The listing builds one solid part. Answer for the finished solid, in the listing's coordinates (mm). A direction names the side the tool comes from. Round coordinates to 2 decimals unless told otherwise and drop trailing zeros. Loops run counter-clockwise (first coordinate to the right, second up) from the corner with the lowest first, then second, coordinate; pieces in that order, holes last. Notation, with made-up numbers: M 62.25,-29 L 119.25,-29 A28 ccw 119.25,-4 Z; hole C 85.5,74 d6. An arc over 180 degrees is marked long. Answer as a JSON object with one key per item and string values.
```python
from build123d import *

# Parameters (mm, degrees)
SKETCH1_R             = 22.225
SKETCH1_R_2           = 20.955
EXTRUDE_THIN1_DEPTH   = 20.32
SKETCH1_R_3           = 14.605
SKETCH1_R_4           = 13.335
EXTRUDE_THIN1_2_DEPTH = 20.32
SKETCH1_3_R           = 8.7757
SKETCH1_3_R_2         = 6.8707
EXTRUDE_THIN2_DEPTH   = 20.32
SKETCH2_W             = 1.27
SKETCH2_H             = 41.91
SKETCH2_W_2           = 41.91
SKETCH2_H_2           = 1.27
EXTRUDE_THIN3_DEPTH   = 20.32
SKETCH1_5_R           = 6.8707
CUT_EXTRUDE1_DEPTH    = 20.32
EXTRUDE_THIN6_DEPTH   = 20.32
CIRPATTERN1_COUNT     = 8


with BuildPart() as part:
    # Sketch1 → Extrude-Thin1 (new body, symmetric)
    with BuildSketch(Plane(origin=(0, 0, 0), x_dir=(0, 0, -1), z_dir=(1, 0, 0))):
        Circle(SKETCH1_R)
        Circle(SKETCH1_R_2, mode=Mode.SUBTRACT)
    extrude(amount=EXTRUDE_THIN1_DEPTH, both=True)



with BuildPart() as body_2:
    # Sketch1 → Extrude-Thin1 2 (new body, symmetric)
    with BuildSketch(Plane(origin=(0, 0, 0), x_dir=(0, 0, -1), z_dir=(1, 0, 0))):
        Circle(SKETCH1_R_3)
        Circle(SKETCH1_R_4, mode=Mode.SUBTRACT)
    extrude(amount=EXTRUDE_THIN1_2_DEPTH, both=True)


with BuildPart() as body_3:
    # Sketch1<3> → Extrude-Thin2 (new body, symmetric)
    with BuildSketch(Plane(origin=(0, 0, 0), x_dir=(0, 0, -1), z_dir=(1, 0, 0))):
        Circle(SKETCH1_3_R)
        Circle(SKETCH1_3_R_2, mode=Mode.SUBTRACT)
    extrude(amount=EXTRUDE_THIN2_DEPTH, both=True)


with BuildPart() as part_1:
    add(part.part)

    add(body_3.part)  # Extrude-Thin3 merges body 3
    # Sketch2 → Extrude-Thin3 (add, symmetric)
    with BuildSketch(Plane(origin=(0, 0, 0), x_dir=(0, 0, -1), z_dir=(1, 0, 0))):
        Rectangle(SKETCH2_W, SKETCH2_H)
        Rectangle(SKETCH2_W_2, SKETCH2_H_2)
        Polygon((-14.368409794, -15.266435406), (15.266435406, 14.368409794), (14.368409794, 15.266435406), (-15.266435406, -14.368409794), align=None)
        Polygon((-15.266435406, 14.368409794), (14.368409794, -15.266435406), (15.266435406, -14.368409794), (-14.368409794, 15.266435406), align=None)
    extrude(amount=EXTRUDE_THIN3_DEPTH, both=True)

    # Sketch1<5> → Cut-Extrude1 (cut, symmetric)
    with BuildSketch(Plane(origin=(0, 0, 0), x_dir=(0, 0, -1), z_dir=(1, 0, 0))):
        Circle(SKETCH1_5_R)
    extrude(amount=CUT_EXTRUDE1_DEPTH, both=True, mode=Mode.SUBTRACT)


    add(body_2.part)  # Extrude-Thin6 merges body 2
    # Sketch4 → Extrude-Thin6 (add, symmetric)
    with BuildSketch(Plane(origin=(0, 0, 0), x_dir=(0, 0, -1), z_dir=(1, 0, 0))):
        Polygon((-8.605794828, 19.116891624), (-5.981351849, 12.78092579), (-4.808024843, 13.266933749), (-7.432467822, 19.602899583), align=None)
    extrude_thin6 = extrude(amount=EXTRUDE_THIN6_DEPTH, both=True)

    # CirPattern1: Extrude-Thin6 ×8 about axis
    cirpattern1_axis = Axis((0, 0, 0), (1, 0, 0))
    for i in range(1, CIRPATTERN1_COUNT):
        add(extrude_thin6.rotate(cirpattern1_axis, i * 360 / CIRPATTERN1_COUNT))


solid = part_1.part
```
Item 1: Flat-ended cylindrical pins translate along their axes: P1, Ø8, axis at y = -3.5, z = 12.5, coming from the +X side; P2, Ø2.5, axis at x = 6.5, z = 10.5, coming from the +Y side; P3, Ø3.5, axis at x = 4.5, y = 11, coming from the -Z side; P4, Ø10, axis at x = 0.5, y = -17.5, coming from the -Z side. Find the tip coordinate at first contact, or state that the pin passes through.
Values follow:
{"P1": "x = 20.32", "P2": "y = 20.21", "P3": "z = -20.21", "P4": "z = -18.38"}
Item 2: The part is cut by section C-C (y = -17). Give the vertices of the cut face in (x, z) (3 decimals), then the cut area to 3 significant figures.
Values follow:
{"outline": "M -20.32,-14.316 L 20.32,-14.316 L 20.32,-12.252 L -20.32,-12.252 Z; M -20.32,-7.729 L 20.32,-7.729 L 20.32,-6.354 L -20.32,-6.354 Z; M -20.32,-0.635 L 20.32,-0.635 L 20.32,0.635 L -20.32,0.635 Z; M -20.32,6.354 L 20.32,6.354 L 20.32,7.729 L -20.32,7.729 Z; M -20.32,12.252 L 20.32,12.252 L 20.32,14.316 L -20.32,14.316 Z", "area": "331 mm^2"}
Item 3: Straight lines are drawn through the part: line 1 (Y direction, x = 11.5, z = 0) (3 decimals); line 2 (Y direction, x = 15, z = -17.5) (3 decimals); line 3 (Z direction, x = -2, y = -3.5). For each, find the intervals that lie inside material, in ascending order.
Values follow:
{"line 1": "-22.225 to -6.871, 6.871 to 22.225", "line 2": "-13.7 to -11.527, -7.936 to -6.561, -0.635 to 0.635, 6.561 to 7.936, 11.527 to 13.7", "line 3": "-21.95 to -20.66, -14.18 to -12.87, -8.05 to -5.91, 5.91 to 8.05, 12.87 to 14.18, 20.66 to 21.95"}
Item 4: Which of the six approach directions +Z, -Z, +X, -X, +Y, -Y give full straight-line access (tool end or side, diameter ignored) to faces 3 (the face through (0.284, 12.126, -8.14)), 4 (the face through (20.32, 7.1, 0))?
Values follow:
{"face 3": "+X, -X", "face 4": "+Z, -Z, +X, +Y, -Y"}
Item 5: The part is cut by section D-D (z = -17.5). Give the vertices of the cut face in (x, y) (3 decimals).
Values follow:
{"outline": "M -20.32,-13.7 L 20.32,-13.7 L 20.32,-11.527 L -20.32,-11.527 Z; M -20.32,-7.936 L 20.32,-7.936 L 20.32,-6.561 L -20.32,-6.561 Z; M -20.32,-0.635 L 20.32,-0.635 L 20.32,0.635 L -20.32,0.635 Z; M -20.32,6.561 L 20.32,6.561 L 20.32,7.936 L -20.32,7.936 Z; M -20.32,11.527 L 20.32,11.527 L 20.32,13.7 L -20.32,13.7 Z"}
Item 6: The part is cut by section A-A (y = 0). Give the vertices of the cut face in (x, z) (3 decimals), then the cut area to 3 significant figures.
Values follow:
{"outline": "M -20.32,-22.225 L 20.32,-22.225 L 20.32,-6.871 L -20.32,-6.871 Z; M -20.32,6.871 L 20.32,6.871 L 20.32,22.225 L -20.32,22.225 Z", "area": "1,250 mm^2"}
Item 7: Determine the mould class of faces 1 (the face through (0.28, 2.82, -14.33)), 2 (the face through (-20.32, 5, 5)) for opening direction Y: released by +Y, released by -Y, zero draft, split by the parting line, or undercut.
Values follow:
{"face 1": "undercut", "face 2": "zero draft"}
